```python
from build123d import *

# Parameters (mm, degrees)
SKETCH1_W           = 27.5
SKETCH1_H           = 18
SKETCH1_R           = 0.75
BOSS_EXTRUDE1_DEPTH = 6
FILLET1_R           = 1
MOVE_FACE1_BY       = 0.08
MOVE_FACE1_2_BY     = 0.08
MOVE_FACE1_3_BY     = 0.08
MOVE_FACE1_4_BY     = 0.08
MOVE_FACE1_5_BY     = 0.08
MOVE_FACE1_6_BY     = 0.08
MOVE_FACE1_7_BY     = 0.08
MOVE_FACE1_8_BY     = 0.08
MOVE_FACE1_9_BY     = 0.08
MOVE_FACE1_10_BY    = 0.08
MOVE_FACE1_11_BY    = 0.08
MOVE_FACE1_12_BY    = 0.08
MOVE_FACE1_13_BY    = 0.08
MOVE_FACE1_14_BY    = 0.08
MOVE_FACE1_15_BY    = 0.08


with BuildPart() as part:
    # Sketch1 → Boss-Extrude1 (new body)
    with BuildSketch(Plane(origin=(0, 0, 0), x_dir=(1, 0, 0), z_dir=(0, 1, 0))):
        with Locations((13.75, 9)):
            Rectangle(SKETCH1_W, SKETCH1_H)
        with Locations(Location((16.5, 7, 0), (0, 0, 270))):
            Circle(SKETCH1_R, mode=Mode.SUBTRACT)
        Polygon((13.656921938, 12), (11.578460969, 15.6), (7.421539031, 15.6), (5.343078062, 12), (7.421539031, 8.4), (11.578460969, 8.4), align=None, mode=Mode.SUBTRACT)
    extrude(amount=BOSS_EXTRUDE1_DEPTH)

    # Fillet1
    fillet1_edges = [part.edges().sort_by_distance(p)[0] for p in [
        (0, 3, -18),
        (27.5, 3, -18),
        (27.5, 3, 0),
        (0, 3, 0),
    ]]
    fillet(fillet1_edges, radius=FILLET1_R)

    # Move Face1: a curved face moved outward by 0.08
    add(Solid.thicken(part.faces().sort_by_distance((16.5, 3, -7.75))[0], MOVE_FACE1_BY))

    # Move Face1 2: a face moved outward by 0.08
    extrude(part.faces().sort_by_distance((12.617691454, 3, -13.8))[0], amount=MOVE_FACE1_2_BY, dir=(-0.866025404, 0, 0.5))

    # Move Face1 3: a face moved outward by 0.08
    extrude(part.faces().sort_by_distance((9.5, 3, -15.6))[0], amount=MOVE_FACE1_3_BY, dir=(0, 0, 1))

    # Move Face1 4: a curved face moved outward by 0.08
    add(Solid.thicken(part.faces().sort_by_distance((27.207106781, 3, -0.292893219))[0], MOVE_FACE1_4_BY))

    # Move Face1 5: a face moved outward by 0.08
    extrude(part.faces().sort_by_distance((27.5, 3, -9))[0], amount=MOVE_FACE1_5_BY, dir=(1, 0, 0))

    # Move Face1 6: a curved face moved outward by 0.08
    add(Solid.thicken(part.faces().sort_by_distance((27.207106781, 3, -17.707106781))[0], MOVE_FACE1_6_BY))

    # Move Face1 7: a face moved outward by 0.08
    extrude(part.faces().sort_by_distance((13.75, 3, -18))[0], amount=MOVE_FACE1_7_BY, dir=(0, 0, -1))

    # Move Face1 8: a curved face moved outward by 0.08
    add(Solid.thicken(part.faces().sort_by_distance((0.292893219, 3, -17.707106781))[0], MOVE_FACE1_8_BY))

    # Move Face1 9: a face moved outward by 0.08
    extrude(part.faces().sort_by_distance((0, 3, -9))[0], amount=MOVE_FACE1_9_BY, dir=(-1, 0, 0))

    # Move Face1 10: a curved face moved outward by 0.08
    add(Solid.thicken(part.faces().sort_by_distance((0.292893219, 3, -0.292893219))[0], MOVE_FACE1_10_BY))

    # Move Face1 11: a face moved outward by 0.08
    extrude(part.faces().sort_by_distance((13.75, 3, 0))[0], amount=MOVE_FACE1_11_BY, dir=(0, 0, 1))

    # Move Face1 12: a face moved outward by 0.08
    extrude(part.faces().sort_by_distance((6.382308546, 3, -13.8))[0], amount=MOVE_FACE1_12_BY, dir=(0.866025404, 0, 0.5))

    # Move Face1 13: a face moved outward by 0.08
    extrude(part.faces().sort_by_distance((9.5, 3, -8.4))[0], amount=MOVE_FACE1_13_BY, dir=(0, 0, -1))

    # Move Face1 14: a face moved outward by 0.08
    extrude(part.faces().sort_by_distance((6.382308546, 3, -10.2))[0], amount=MOVE_FACE1_14_BY, dir=(0.866025404, 0, -0.5))

    # Move Face1 15: a face moved outward by 0.08
    extrude(part.faces().sort_by_distance((12.617691454, 3, -10.2))[0], amount=MOVE_FACE1_15_BY, dir=(-0.866025404, 0, -0.5))


solid = part.part
```
Design review of the part built by this model. Coordinates are the model's own, in mm. A direction names the side the tool comes from. Coordinates: 2 decimals unless noted, no trailing zeros. Loops run counter-clockwise (first coordinate to the right, second up) from the corner with the lowest first, then second, coordinate; pieces in that order, holes last.
Q1. Tool access review of faces 4 (the face through (0.23, 3.04, -17.76)), 5 (the face through (6.466, 2.958, -13.785)): name each direction out of +Z, -Z, +X, -X, +Y, -Y from which nothing blocks a thin tool from reaching the whole face with its end or side.
Reported:
face 4: -Z, -X, +Y, -Y
face 5: +Y, -Y
Q2. We need section C-C on y = 1. State the section outline as (x, z) points, and give its area (3 significant figures).
Reported:
outline: (-0.08, -17) arc R1.08 ccw to (1, -18.08) - (26.5, -18.08) arc R1.08 ccw to (27.58, -17) - (27.58, -1) arc R1.08 ccw to (26.5, 0.08) - (1, 0.08) arc R1.08 ccw to (-0.08, -1) - close; hole (5.44, -12) - (7.47, -15.52) - (11.53, -15.52) - (13.56, -12) - (11.53, -8.48) - (7.47, -8.48) - close; hole circle Ø1.34 at (16.5, -7)
area: 457 mm2
Q3. To check wall thickness, follow line 1 (Z direction, x = 11.5, y = 5.2); line 2 (X direction, y = 3.9, z = -7); line 3 (X direction, y = 5.05, z = -9.25). State the ranges of each line that lie inside material, in increasing order.
Reported:
line 1: z = -18.08 to -15.52, -8.48 to 0.08
line 2: x = -0.08 to 15.83, 17.17 to 27.58
line 3: x = -0.08 to 7.02, 11.98 to 27.58
Q4. We need section B-B on z = -7. State the section outline as (x, y) points, and give its area (3 significant figures).
Reported:
outline: (-0.08, 0) - (15.83, 0) - (15.83, 6) - (-0.08, 6) - close; (17.17, 0) - (27.58, 0) - (27.58, 6) - (17.17, 6) - close
area: 158 mm2
Q5. We need section A-A on x = 10. State the section outline as (y, z) points, and give its area (3 significant figures).
Reported:
outline: (0, -18.08) - (6, -18.08) - (6, -15.52) - (0, -15.52) - close; (0, -8.48) - (6, -8.48) - (6, 0.08) - (0, 0.08) - close
area: 66.7 mm2
Q6. The part is to be moulded in two halves that separate along Z. For faces 1 (the face through (14, 3, 0.08)), 2 (the face through (17.065, 2.958, -6.64)), 3 (the face through (27.26, 3.04, -17.77)), say which applies: +Z half, -Z half, draft (parallel to the pull), parting line (faces both ways), or undercut.
Reported:
face 1: +Z half
face 2: undercut
face 3: -Z half
Q7. For pin 1 (0.8 mm diameter, centred on x = 16.5, z = -7, fed in from -Y), flat-tipped, find the tip position at first contact; note if it passes through.
Reported:
pin 1: passes through
